Check sheet for the modelled part. Datum: model origin and axes. Units: mm. A direction names the side the tool comes from. Round coordinates to 2 decimals unless told otherwise and drop trailing zeros. Loops run counter-clockwise (first coordinate to the right, second up) from the corner with the lowest first, then second, coordinate; pieces in that order, holes last. Notation, with made-up numbers: (-33.75, -9.5) - (13.25, -9.5) arc R18 cw to (13.25, 17.5) - close; hole circle Ø6 at (-4, 39.25). An arc over 180 degrees is marked (long way). Return JSON: item names as keys, results as strings.
from build123d import *

# Parameters (mm, degrees)
F0_R     = 38.5
F2_DEPTH = 5
F0_R_2   = 41.5
F1_W     = 2
F1_H     = 74.3572457801
F3_DEPTH = 80
F5_DEPTH = 3
F6_R     = 0.99999


# Not quite as in the source:
# - a fillet or chamfer is up to 0.001 mm smaller than in the source, because OpenCascade refuses the exact size


with BuildPart() as f2:
    # F0 (on Top) → F2 (new body)
    with BuildSketch(Plane.XY):
        Circle(F0_R)
    extrude(amount=F2_DEPTH)

    # F0 (on Top) + F1 (on Top) → F3 (join)
    with BuildSketch(Plane.XY):
        Circle(F0_R_2)
        Circle(F0_R, mode=Mode.SUBTRACT)
    with BuildSketch(Plane.XY):
        with Locations((11, 0)):
            Rectangle(F1_W, F1_H)
    extrude(amount=F3_DEPTH)

    # F4 (on Top) → F5 (cut)
    with BuildSketch(Plane.XY):
        Polygon((0, -3), (-4, -38), (4, -38), align=None)
        Polygon((15.5468718514, -34.9040796417), (0.9270509831, -2.8531695489), (7.9384197211, -37.3762155967), align=None)
        Polygon((25.5719075646, -28.3915047771), (1.7633557569, -2.4270509831), (19.0997716096, -33.0937867954), align=None)
        Polygon((33.0937867954, -19.0997716096), (2.4270509831, -1.7633557569), (28.3915047771, -25.5719075646), align=None)
        Polygon((37.3762155967, -7.9384197211), (2.8531695489, -0.9270509831), (34.9040796417, -15.5468718514), align=None)
        Polygon((38, 4), (3, 0), (38, -4), align=None)
        Polygon((34.9040796417, 15.5468718514), (2.8531695489, 0.9270509831), (37.3762155967, 7.9384197211), align=None)
        Polygon((28.3915047771, 25.5719075646), (2.4270509831, 1.7633557569), (33.0937867954, 19.0997716096), align=None)
        Polygon((19.0997716096, 33.0937867954), (1.7633557569, 2.4270509831), (25.5719075646, 28.3915047771), align=None)
        Polygon((7.9384197211, 37.3762155967), (0.9270509831, 2.8531695489), (15.5468718514, 34.9040796417), align=None)
        Polygon((-4, 38), (0, 3), (4, 38), align=None)
        Polygon((-15.5468718514, 34.9040796417), (-0.9270509831, 2.8531695489), (-7.9384197211, 37.3762155967), align=None)
        Polygon((-25.5719075646, 28.3915047771), (-1.7633557569, 2.4270509831), (-19.0997716096, 33.0937867954), align=None)
        Polygon((-33.0937867954, 19.0997716096), (-2.4270509831, 1.7633557569), (-28.3915047771, 25.5719075646), align=None)
        Polygon((-37.3762155967, 7.9384197211), (-2.8531695489, 0.9270509831), (-34.9040796417, 15.5468718514), align=None)
        Polygon((-38, -4), (-3, 0), (-38, 4), align=None)
        Polygon((-34.9040796417, -15.5468718514), (-2.8531695489, -0.9270509831), (-37.3762155967, -7.9384197211), align=None)
        Polygon((-28.3915047771, -25.5719075646), (-2.4270509831, -1.7633557569), (-33.0937867954, -19.0997716096), align=None)
        Polygon((-19.0997716096, -33.0937867954), (-1.7633557569, -2.4270509831), (-25.5719075646, -28.3915047771), align=None)
        Polygon((-7.9384197211, -37.3762155967), (-0.9270509831, -2.8531695489), (-15.5468718514, -34.9040796417), align=None)
    extrude(amount=F5_DEPTH, mode=Mode.SUBTRACT)

    # F6 (radius 1 in the source; OpenCascade refuses exactly that, so slightly less here)
    f6_edges = [f2.edges().sort_by_distance(p)[0] for p in [
        (-38.5, 0, 80),
        (-41.5, 0, 80),
        (12, 0, 80),
        (10, 0, 80),
        (38.5, 0, 80),
    ]]
    fillet(f6_edges, radius=F6_R)


solid = f2.part
Q1. Sectioned sample at A-A (z = 74). Enter the section's corners in (x, y), plus the area to 3 significant figures.
Answer key:
{"outline": "circle Ø83 at (0, 0); hole (10, -37.18) - (10, 37.18) arc R38.5 ccw (long way) to start; hole (12, -36.58) arc R38.5 ccw to (12, 36.58) - close", "area": "902 mm²"}
Q2. Draft check along X on faces 1 (the face through (10.31, -17.546, 1.479)), 2 (the face through (9, -39, 80)). Enter one of: released by +X, released by -X, zero draft, split by the parting line, or undercut.
Answer key:
{"face 1": "undercut", "face 2": "zero draft"}
Q3. Depth check by flat-ended pin: P1, Ø2.5, axis at y = -1.5, z = 1, coming from the +X side; P2, Ø7, axis at x = 12, y = -18.5, coming from the -Z side; P3, Ø2, axis at x = -1, y = -32.5, coming from the +Z side; P4, Ø5, axis at y = -23, z = 40, coming from the +X side. Enter the tip coordinate at first touch or a pass-through.
Answer key:
{"P1": "stops at x = 41.5", "P2": "stops at z = 0", "P3": "stops at z = 5", "P4": "stops at x = 36.08"}
Q4. Scan lines: probe 1 along Y at (x, z) = (0, 61); probe 2 along X at (y, z) = (33.5, 53); probe 3 along X at (y, z) = (-9.5, 30). Record each from-to range of solid material in increasing order. Write a range as [from, to].
Answer key:
{"probe 1": "y = [-41.5, -38.5], [38.5, 41.5]", "probe 2": "x = [-24.49, -18.97], [10, 12], [18.97, 24.49]", "probe 3": "x = [-40.4, -37.31], [10, 12], [37.31, 40.4]"}
Q5. Tool access check on faces 3 (the face through (-22.38, -30.71, 1.48)), 4 (the face through (-38.487, 0.988, 41.482)). Record the directions out of +Z, -Z, +X, -X, +Y, -Y that give a thin tool (end or side, any length) a straight path to the whole face; none if there is none.
Answer key:
{"face 3": "-Z", "face 4": "+Z"}
